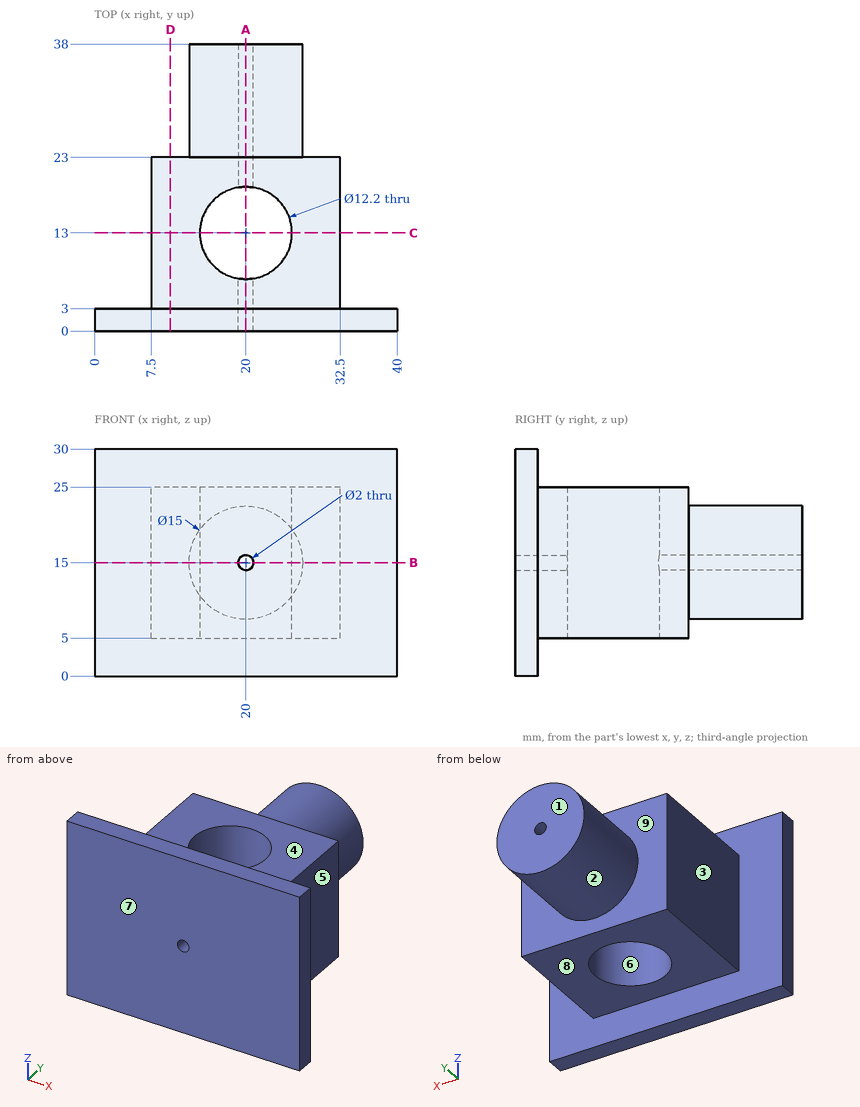
Check sheet for the drawn part. Datum: minimum x, y, z corner. Units: mm. A direction names the side the tool comes from. Give positions to 0.01 mm unless a question says otherwise; leave off trailing zeros. Write each loop counter-clockwise with the first axis right and the second up, starting at its lowest first coordinate (ties: lowest second). Pieces come first, ordered by that corner, then holes. Notation, with made-up numbers: M 80.5,-39 L 132.5,-39 A32 cw 132.5,-5 Z; hole C 19.25,32.5 d10. An arc over 180 degrees is marked long. Write item = value, one per line.
(1) Sectioned sample at D-D (x = 10). Record the cut outline in (y, z), then the cut area to 3 significant figures.
Found:
outline = M 0,0 L 3,0 L 3,5 L 23,5 L 23,25 L 3,25 L 3,30 L 0,30 Z
area = 490 mm2
(2) Sectioned sample at C-C (y = 13). Record the cut outline in (x, z).
Found:
outline = M 7.5,5 L 13.9,5 L 13.9,25 L 7.5,25 Z; M 26.1,5 L 32.5,5 L 32.5,25 L 26.1,25 Z
(3) Go/stop test with flat-tipped pins: pin 1 Ø10 at (x, y) = (22, 9) entering from -Z; pin 2 Ø1 at (x, z) = (10.5, 5.5) entering from +Y; pin 3 Ø12 at (y, z) = (17, 13) entering from +X; pin 4 Ø22 at (x, y) = (20.5, 13) entering from +Z. Record where each tip stops, or that it passes through.
Found:
pin_1 = 5
pin_2 = 23
pin_3 = 32.5
pin_4 = 30
(4) Material ranges on line 1 (Y direction, x = 20, z = 9.5); line 2 (Z direction, x = 20, y = 31.5); line 3 (X direction, y = 34.25, z = 15), recorded low to high.
Found:
line_1 = 0 to 6.9, 19.1 to 38
line_2 = 7.5 to 14, 16 to 22.5
line_3 = 12.5 to 19, 21 to 27.5
(5) Draft check along Y on the marked faces 6, 7, 8 and 9. Enter one of: released by +Y, released by -Y, zero draft, split by the parting line, or undercut.
Found:
face_6 = undercut
face_7 = released by -Y
face_8 = zero draft
face_9 = released by +Y
(6) Access from +Z, -Z, +X, -X, +Y, -Y to the whole of each face (thin tool, end or side, straight path). Record for the marked faces 1, 2, 3, 4 and 5.
Found:
face_1 = +Z, -Z, +X, -X, +Y
face_2 = +Y
face_3 = +Z, -Z, -X, +Y
face_4 = +Z, +X, -X, +Y
face_5 = +Z, -Z, +X, +Y
(7) Sectioned sample at B-B (z = 15). Record the cut outline in (x, y).
Found:
outline = M 0,0 L 19,0 L 19,6.98 A6.1 cw 19,19.02 L 19,38 L 12.5,38 L 12.5,23 L 7.5,23 L 7.5,3 L 0,3 Z; M 21,0 L 40,0 L 40,3 L 32.5,3 L 32.5,23 L 27.5,23 L 27.5,38 L 21,38 L 21,19.02 A6.1 cw 21,6.98 Z
(8) Sectioned sample at A-A (x = 20). Record the cut outline in (y, z), then the cut area to 3 significant figures.
Found:
outline = M 0,0 L 3,0 L 3,5 L 6.9,5 L 6.9,14 L 0,14 Z; M 0,16 L 6.9,16 L 6.9,25 L 3,25 L 3,30 L 0,30 Z; M 19.1,5 L 23,5 L 23,7.5 L 38,7.5 L 38,14 L 19.1,14 Z; M 19.1,16 L 38,16 L 38,22.5 L 23,22.5 L 23,25 L 19.1,25 Z
area = 419 mm2
